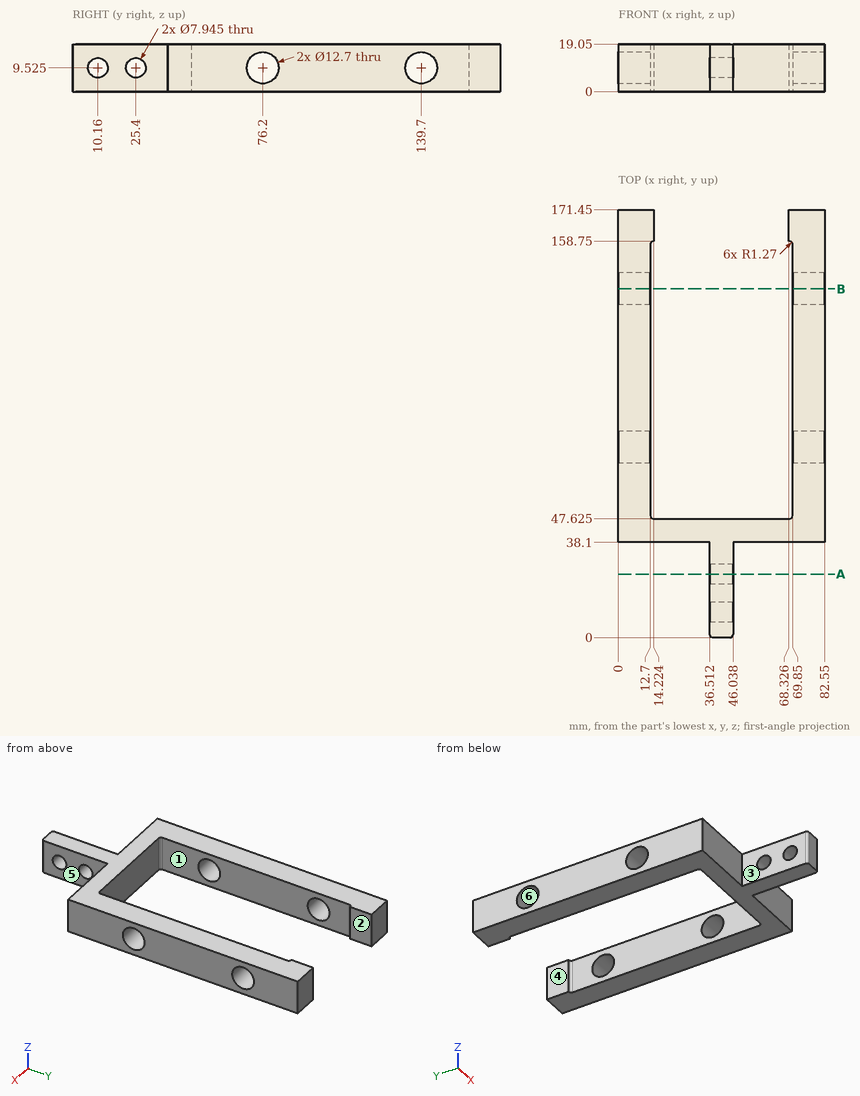
The drawing under review shows one solid part. Ordinate dimensions are in mm from its lowest x, y, z. A direction names the side the tool comes from. Give positions to 0.01 mm unless a question says otherwise; leave off trailing zeros. Order: outer loops, then holes, each group sorted by start corner. A loop starts at its lowest first (then second) coordinate and runs counter-clockwise, first axis right, second up. Notation, with made-up numbers: M 72,1.5 L 78,1.5 A27 ccw 78,17.5 Z; hole C 30.5,-35 d9. An arc over 180 degrees is marked long. One line per question, with ' | ' between items. Start each with the question number.
Q1. The part is to be moulded in two halves that separate along X. For the marked faces 4, 5 and 6, say which applies: +X half, -X half, draft (parallel to the pull), parting line (faces both ways), or undercut.
Q2. We need section B-B (y = 139.7). State how many separate pieces and enclosed holes the cut face has, plus the area to 3 significant figures.
Q3. For L1, parallel to X at y = 67.5, z = 5.75; L2, parallel to Z at x = 72, y = 76; L3, parallel to Y at x = 31.5, z = 15.75 (1 decimal), list the stretches that pass through material, from the lowest coordinate up. Write a range as [from, to].
Q4. Machinability: for the marked faces 1, 2 and 3, which of the approach directions +Z, -Z, +X, -X, +Y, -Y give a long, thin tool a straight path to every point of the face, cutting with its end or side? Answer none if there is none.
Q5. We need section A-A (y = 25.4). Write out the cut boundary in (x, z).
Q6. For pin 1 Ø10 at (x, z) = (30.5, 14.5) entering from +Y (1 decimal); pin 2 Ø9 at (y, z) = (25.4, 9.525) entering from -X; pin 3 Ø3 at (x, y) = (68.5, 48.5) entering from +Z; pin 4 Ø1 at (x, z) = (20.5, 8.5) entering from -Y, all flat-tipped, find the tip position at first contact; note any pin that passes through.
Returned:
1) face 4: undercut | face 5: +X half | face 6: draft
2) separate pieces: 4 | enclosed holes: 0 | area: 161 mm2
3) L1: [0, 12.7], [69.85, 82.55] | L2: [0, 3.18], [15.87, 19.05] | L3: [38.1, 47.6]
4) face 1: +Z, -Z | face 2: +Z, -Z, +Y | face 3: +Z, -Z, -X, -Y
5) outline: M 36.51,0 L 46.04,0 L 46.04,5.55 L 36.51,5.55 Z; M 36.51,13.5 L 46.04,13.5 L 46.04,19.05 L 36.51,19.05 Z
6) pin 1: y = 47.6 | pin 2: x = 36.51 | pin 3: z = 19.05 | pin 4: y = 38.1
